```python
from build123d import *

# Parameters (mm, degrees)
SKETCH1_R                                = 155
BOSS_EXTRUDE1_DEPTH                      = 15
CBORE_FOR_M10_HEX_HEAD_BOLT1_D           = 10.5
CBORE_FOR_M10_HEX_HEAD_BOLT1_CBORE_D     = 21.48
CBORE_FOR_M10_HEX_HEAD_BOLT1_CBORE_DEPTH = 6.85
CIRPATTERN1_COUNT                        = 8
SKETCH2_R                                = 40
CUT_EXTRUDE1_DEPTH                       = 15
FILLET1_R                                = 5


with BuildPart() as part:
    # Sketch1 → Boss-Extrude1 (new body)
    with BuildSketch(Plane(origin=(0, 0, 0), x_dir=(1, 0, 0), z_dir=(0, 1, 0))):
        with Locations(Location((0, 0, 0), (0, 0, 270))):
            Circle(SKETCH1_R)
    extrude(amount=BOSS_EXTRUDE1_DEPTH)

    # CBORE for M10 Hex Head Bolt1 (through all)
    with Locations(Plane(origin=(0, 15, -137.5), x_dir=(0, 0, 1), z_dir=(0, 1, 0))):
        with Locations((0, 0)):
            cbore_for_m10_hex_head_bolt1 = CounterBoreHole(CBORE_FOR_M10_HEX_HEAD_BOLT1_D / 2, CBORE_FOR_M10_HEX_HEAD_BOLT1_CBORE_D / 2, CBORE_FOR_M10_HEX_HEAD_BOLT1_CBORE_DEPTH)

    # CirPattern1: CBORE for M10 Hex Head Bolt1 ×8 about axis
    cirpattern1_axis = Axis((0, 0, 0), (0, 1, 0))
    for i in range(1, CIRPATTERN1_COUNT):
        add(cbore_for_m10_hex_head_bolt1.rotate(cirpattern1_axis, i * 360 / CIRPATTERN1_COUNT), mode=Mode.SUBTRACT)

    # Sketch2 → Cut-Extrude1 (cut)
    with BuildSketch(Plane(origin=(0, 15, 0), x_dir=(1, 0, 0), z_dir=(0, 1, 0))):
        with Locations(Location((0, 0, 0), (0, 0, 270))):
            Circle(SKETCH2_R)
    extrude(amount=-CUT_EXTRUDE1_DEPTH, mode=Mode.SUBTRACT)

    # Fillet1
    fillet1_edges = [part.edges().sort_by_distance(p)[0] for p in [
        (0, 15, -155),
    ]]
    fillet(fillet1_edges, radius=FILLET1_R)


solid = part.part
```
Read the model definition and answer for the solid it produces. Units are mm, in the model's axes. A direction names the side the tool comes from. Round coordinates to 2 decimals unless told otherwise and drop trailing zeros. One line per item, written item: value.
1) A cutting plane is placed at A-A (y = 4.25). Give the number of separate pieces and of enclosed holes in the cut face, and give its area (3 significant figures).
Answer list:
separate pieces: 1
enclosed holes: 9
area: 69,800 mm²
2) Consider L1, parallel to X at y = 10.5, z = 94.5; L2, parallel to Z at x = 105.5, y = 12.75; L3, parallel to X at y = 2.75, z = 97. Determine where each line is inside the solid, lowest interval first. Write a range as [from, to].
Answer list:
L1: x = [-122.83, -107.62], [-86.84, 86.84], [107.62, 122.83]
L2: z = [-112.43, -104.08], [-90.38, 90.38], [104.08, 112.43]
L3: x = [-120.9, -102.47], [-91.98, 91.98], [102.47, 120.9]
3) The mould has two halves that part along Z. Classify faces 3 (the face through (-99.653, 4.018, -101.883)), 4 (the face through (-32, 0, 32)): pulls with the +Z half, pulls with the -Z half, needs draft (parallel to the pull), parting line crosses it, or undercut.
Answer list:
face 3: undercut
face 4: needs draft
4) For faces 1 (the face through (105.75, 11.62, -90.69)), 2 (the face through (-142.5, 4, -1.6)), determine the directions among +Z, -Z, +X, -X, +Y, -Y from which every point of the face is accessible in a straight line to the end or side of a thin tool.
Answer list:
face 1: +Y
face 2: +Y, -Y
5) Flat-ended cylindrical pins translate along their axes: P1, Ø3, axis at x = -44, y = 5.5, coming from the +Z side; P2, Ø2, axis at x = 105.5, y = 8, coming from the -Z side; P3, Ø3, axis at x = 26.5, y = 2, coming from the -Z side; P4, Ø23.5, axis at x = -98.5, z = 95.5, coming from the +Y side. Find the tip coordinate at first contact, or state that the pin passes through.
Answer list:
P1: stops at z = 149.06
P2: stops at z = -114.48
P3: stops at z = -152.97
P4: stops at y = 15
